```python
from build123d import *

# Parameters (mm, degrees)
SKETCH_1_W             = 63
SKETCH_1_H             = 40.3
EXTRUDE_1_DEPTH        = 2
CUT_EXTRUDE_1_REACH    = 39.447
SKETCH_2_R             = 1.5
FILLET_1_R             = 3
SKETCH_3_W             = 41
SKETCH_3_H             = 5
SKETCH_3_W_2           = 28
EXTRUDE_2_DEPTH        = 10
SKETCH_4_W             = 12
SKETCH_4_H             = 27
EXTRUDE_3_DEPTH        = 10
CUT_EXTRUDE_2_REACH    = 69.224
SKETCH_5_W             = 2
SKETCH_5_H             = 5
PATTERN_LINEAR_1_COUNT = 5
PATTERN_LINEAR_1_PITCH = 5
SKETCH_6_R             = 0.2
EXTRUDE_4_DEPTH        = 10
PATTERN_LINEAR_2_COUNT = 8
PATTERN_LINEAR_2_PITCH = 2.54


with BuildPart() as part:
    # 草图1 → 凸台-拉伸1 (new body)
    with BuildSketch(Plane(origin=(0, 0, 0), x_dir=(1, 0, 0), z_dir=(0, 1, 0))):
        Rectangle(SKETCH_1_W, SKETCH_1_H)
    extrude(amount=EXTRUDE_1_DEPTH)

    # 草图2 → 切除-拉伸1 (cut, up to next)
    with BuildSketch(Plane(origin=(0, 2, 0), x_dir=(1, 0, 0), z_dir=(0, 1, 0)), mode=Mode.PRIVATE) as cut_extrude_1_sk1:
        with Locations(Location((-26.5, 15.15, 0), (0, 0, 270))):
            Circle(SKETCH_2_R)
    cut_extrude_1_tool1 = extrude(cut_extrude_1_sk1.sketch, amount=-CUT_EXTRUDE_1_REACH, mode=Mode.PRIVATE) & part.part
    # 草图2 → 切除-拉伸1 (cut, up to next)
    with BuildSketch(Plane(origin=(0, 2, 0), x_dir=(1, 0, 0), z_dir=(0, 1, 0)), mode=Mode.PRIVATE) as cut_extrude_1_sk2:
        with Locations(Location((25.98, -14.27, 0), (0, 0, 270))):
            Circle(SKETCH_2_R)
    cut_extrude_1_tool2 = extrude(cut_extrude_1_sk2.sketch, amount=-CUT_EXTRUDE_1_REACH, mode=Mode.PRIVATE) & part.part
    add(cut_extrude_1_tool1.solids().sort_by_distance((-26.5, 2, -15.15))[0], mode=Mode.SUBTRACT)
    add(cut_extrude_1_tool2.solids().sort_by_distance((25.98, 2, 14.27))[0], mode=Mode.SUBTRACT)

    # 圆角1
    fillet_1_edges = [part.edges().sort_by_distance(p)[0] for p in [
        (31.5, 1, 20.15),
        (-31.5, 1, 20.15),
        (-31.5, 1, -20.15),
        (31.5, 1, -20.15),
    ]]
    fillet(fillet_1_edges, radius=FILLET_1_R)

    # 草图3 → 凸台-拉伸2 (add)
    with BuildSketch(Plane(origin=(0, 0, 0), x_dir=(-1, 0, 0), z_dir=(0, -1, 0))):
        with Locations((0, 13.65)):
            Rectangle(SKETCH_3_W, SKETCH_3_H)
        with Locations((-2.5, -13.65)):
            Rectangle(SKETCH_3_W_2, SKETCH_3_H)
    extrude(amount=EXTRUDE_2_DEPTH)

    # 草图4 → 凸台-拉伸3 (add)
    with BuildSketch(Plane(origin=(0, 2, 0), x_dir=(1, 0, 0), z_dir=(0, 1, 0))):
        with Locations((-25.5, -3.65)):
            Rectangle(SKETCH_4_W, SKETCH_4_H)
    extrude(amount=EXTRUDE_3_DEPTH)

    # 草图5 → 切除-拉伸2 (cut, up to next)
    with BuildSketch(Plane.ZY.offset(31.5), mode=Mode.PRIVATE) as cut_extrude_2_sk1:
        with Locations((-6.85, 7.5)):
            Rectangle(SKETCH_5_W, SKETCH_5_H)
    cut_extrude_2_tool1 = extrude(cut_extrude_2_sk1.sketch, amount=-CUT_EXTRUDE_2_REACH, mode=Mode.PRIVATE) & part.part
    cut_extrude_2 = cut_extrude_2_tool1.solids().sort_by_distance((-31.5, 7.5, -6.85))[0]
    add(cut_extrude_2, mode=Mode.SUBTRACT)

    # 阵列(线性)1: 切除-拉伸2 ×5
    with Locations(*[(0, 0, i * PATTERN_LINEAR_1_PITCH) for i in range(1, PATTERN_LINEAR_1_COUNT)]):
        add(cut_extrude_2, mode=Mode.SUBTRACT)

    # 草图6 → 凸台-拉伸4 (add)
    with BuildSketch(Plane(origin=(0, 2, 0), x_dir=(1, 0, 0), z_dir=(0, 1, 0))):
        with Locations(Location((26.5, 15.15, 0), (0, 0, 90))):
            Circle(SKETCH_6_R)
    extrude_4 = extrude(amount=EXTRUDE_4_DEPTH)

    # 阵列(线性)2: 凸台-拉伸4 ×8
    with Locations(*[(0, 0, i * PATTERN_LINEAR_2_PITCH) for i in range(1, PATTERN_LINEAR_2_COUNT)]):
        add(extrude_4)


solid = part.part
```
Check sheet for the modelled part. Datum: model origin and axes. Units: mm. A direction names the side the tool comes from. Give positions to 0.01 mm unless a question says otherwise; leave off trailing zeros. Write each loop counter-clockwise with the first axis right and the second up, starting at its lowest first coordinate (ties: lowest second). Pieces come first, ordered by that corner, then holes. Notation, with made-up numbers: (47, 72.5) - (58, 72.5) arc R11 ccw to (58, 87.5) - close; hole circle Ø9 at (5, 39.5). An arc over 180 degrees is marked (long way). Answer as a JSON object with one key per item and string values. Group by question number.
1) Sectioned sample at B-B (z = 8). Record the cut outline in (x, y), then the cut area to 3 significant figures.
2) Depth check by flat-ended pin: P1, Ø4, axis at x = -27.5, y = 7.5, coming from the +Z side; P2, Ø0.6, axis at x = -25.5, z = 8, coming from the -Y side; P3, Ø1.5, axis at y = -7, z = 12.5, coming from the -X side; P4, Ø5, axis at x = -25, y = -5.5, coming from the +Z side. Enter the tip coordinate at first touch or a pass-through.
3) Sectioned sample at D-D (x = -16). Record the cut outline in (y, z).
4) Access from +Z, -Z, +X, -X, +Y, -Y to the whole of each face (thin tool, end or side, straight path). Record for faces 1 (the face through (-26, 10, -2)), 2 (the face through (-26, 7, -0.85)), 3 (the face through (16.5, -5, 14)), 4 (the face through (0, -5, -11.15)).
5) Sectioned sample at A-A (x = -26.5). Give the number of separate pieces and of enclosed holes in the cut face, then the cut area to 3 significant figures.
6) Thickness scan on probe 1 along Z at (x, y) = (-26.5, 5.75); probe 2 along Y at (x, z) = (-27.5, 7.5); probe 3 along X at (y, z) = (1.45, -15.15). Record the ranges inside material, lowest first. Write a range as from..to.
7) Release check for a two-part mould opening along Y. For faces 5 (the face through (-26, 10, 13)), 6 (the face through (31.5, 1, 0)), 7 (the face through (3, -10, 14)) record: pulls with the +Y half, pulls with the -Y half, needs draft (parallel to the pull), parting line crosses it, or undercut.
Geometry results:
{
 "1": {"outline": "(-31.5, 0) - (31.5, 0) - (31.5, 2) - (-19.5, 2) - (-19.5, 5) - (-31.5, 5) - close; (-31.5, 10) - (-19.5, 10) - (-19.5, 12) - (-31.5, 12) - close", "area": "186 mm^2"},
 "2": {"P1": "stops at z = 17.15", "P2": "stops at y = 0", "P3": "stops at x = -11.5", "P4": "passes through"},
 "3": {"outline": "(-10, -16.15) - (0, -16.15) - (0, -20.15) - (2, -20.15) - (2, 20.15) - (0, 20.15) - (0, -11.15) - (-10, -11.15) - close"},
 "4": {"face 1": "-X", "face 2": "+X, -X", "face 3": "+Z, +X, -Y", "face 4": "+X, -X, -Y"},
 "5": {"separate pieces": "2", "enclosed holes": "5", "area": "295 mm^2"},
 "6": {"probe 1": "z = -9.85..-7.85, -5.85..-2.85, -0.85..2.15, 4.15..7.15, 9.15..12.15, 14.15..17.15", "probe 2": "y = 0..5, 10..12", "probe 3": "x = -31.5..-28, -25..31.5"},
 "7": {"face 5": "undercut", "face 6": "needs draft", "face 7": "pulls with the -Y half"}
}
